Could you check a few things on this model? Use its own coordinates, in mm. A direction names the side the tool comes from. Round coordinates to 2 decimals unless told otherwise and drop trailing zeros. Loops run counter-clockwise (first coordinate to the right, second up) from the corner with the lowest first, then second, coordinate; pieces in that order, holes last. Notation, with made-up numbers: (68.25, -6) - (84.25, -6) arc R23 ccw to (84.25, 27) - close; hole circle Ø5 at (-36, -12.75). An arc over 180 degrees is marked (long way). Answer as CSV lines item,"result". Start each with the question number.
1) Suppose I cut it at D-D, the plane x = 17.05. Write out the boundary of the cut face in (y, z), then the cut area to 3 significant figures.
2) Please list where these lines run through material, in increasing order: line 1 along Y through (x, z) = (17.05, 9); line 2 along Y through (x, z) = (90.25, 10); line 3 along Y through (x, z) = (5, 11.5).
3) Which directions (+Z, -Z, +X, -X, +Y, -Y) give clear straight access to the entire face, cutting with the end or side of a thin tool? Please do faces 5 (the face through (48.31, 26.7, 7.28)), 6 (the face through (13, 13.25, 7)).
4) Suppose I cut it at A-A, the plane x = 90.25. Write out the boundary of the cut face in (y, z), then the cut area to 3 significant figures.
5) Suppose I cut it at C-C, the plane y = -27.5. Write out the boundary of the cut face in (x, z), then the cut area to 3 significant figures.
6) Suppose I cut it at B-B, the plane z = 9.5. Count the separate pieces of the cut face and the enclosed holes in it, then the cut area to 3 significant figures.
7) I'm going to push flat-ended pins straight in: pin 1 Ø1.5 at (x, z) = (23.5, 4.5) entering from +Y; pin 2 Ø2 at (x, z) = (27.5, 5.5) entering from +Y. Where does each tip first touch, or does it pass through?
8) We'd pull the mould along Y, two halves only. Please class faces 1 (the face through (13, -13.25, 7)), 2 (the face through (49.3, 37.215, 4.465)), 3 (the face through (0, 29, 7)), 4 (the face through (24, -12.2, 7.4)): pulls with the +Y half, pulls with the -Y half, needs draft (parallel to the pull), parting line crosses it, or undercut.
```python
from build123d import *

# Parameters (mm, degrees)
BOSS_EXTRUDE1_DEPTH         = 12.7
CHAMFER1_SIZE               = 5
FILLET1_R                   = 3.5
TAP_DRILL_FOR_M5X0_8_TAP1_D = 4.2
CUT_EXTRUDE1_DEPTH          = 2
CHAMFER3_SIZE               = 5
TAP_DRILL_FOR_M4X0_7_TAP1_D = 3.3
CUT_EXTRUDE2_DEPTH          = 2


with BuildPart() as part:
    # Sketch1 → Boss-Extrude1 (new body)
    with BuildSketch(Plane.XY):
        with BuildLine():
            Line((0, 38.75), (0, 13.25))
            Line((0, 13.25), (25, 13.25))
            Line((25, 13.25), (25, -13.25))
            Line((25, -13.25), (0, -13.25))
            Line((0, -13.25), (0, -38.75))
            ThreePointArc((0, -38.75), (0.292893219, -39.457106781), (1, -39.75))
            Line((1, -39.75), (99, -39.75))
            ThreePointArc((99, -39.75), (99.707106781, -39.457106781), (100, -38.75))
            Line((100, -38.75), (100, 38.75))
            ThreePointArc((100, 38.75), (99.707106781, 39.457106781), (99, 39.75))
            Line((99, 39.75), (1, 39.75))
            ThreePointArc((1, 39.75), (0.292893219, 39.457106781), (0, 38.75))
        make_face()
    extrude(amount=BOSS_EXTRUDE1_DEPTH)

    # Chamfer1
    chamfer1_edges = [part.edges().sort_by_distance(p)[0] for p in [
        (0, 13.25, 6.35),
        (0, -13.25, 6.35),
    ]]
    chamfer(chamfer1_edges, length=CHAMFER1_SIZE)

    # Fillet1
    fillet1_edges = [part.edges().sort_by_distance(p)[0] for p in [
        (25, -13.25, 6.35),
        (25, 13.25, 6.35),
    ]]
    fillet(fillet1_edges, radius=FILLET1_R)

    # Tap Drill for M5x0.8 Tap1 (through all)
    with Locations(Plane.XY.offset(12.7)):
        with Locations((10.25, 27.5), (50.25, 27.5), (90.25, 27.5), (90.25, -27.5), (50.25, -27.5), (10.25, -27.5)):
            Hole(TAP_DRILL_FOR_M5X0_8_TAP1_D / 2)

    # Sketch8 → Cut-Extrude1 (cut)
    with BuildSketch(Plane(origin=(0, 0, 0), x_dir=(-1, 0, 0), z_dir=(0, 0, -1))):
        with BuildLine():
            Line((-21.5, 13.25), (-5, 13.25))
            Line((-5, 13.25), (0, 18.25))
            Line((0, 18.25), (0, 38.75))
            ThreePointArc((0, 38.75), (-0.292893219, 39.457106781), (-1, 39.75))
            Line((-1, 39.75), (-99, 39.75))
            ThreePointArc((-99, 39.75), (-99.707106781, 39.457106781), (-100, 38.75))
            Line((-100, 38.75), (-100, -38.75))
            ThreePointArc((-100, -38.75), (-99.707106781, -39.457106781), (-99, -39.75))
            Line((-99, -39.75), (-1, -39.75))
            ThreePointArc((-1, -39.75), (-0.292893219, -39.457106781), (0, -38.75))
            Line((0, -38.75), (0, -18.25))
            Line((0, -18.25), (-5, -13.25))
            Line((-5, -13.25), (-21.5, -13.25))
            ThreePointArc((-21.5, -13.25), (-23.974873734, -12.224873734), (-25, -9.75))
            Line((-25, -9.75), (-25, 9.75))
            ThreePointArc((-25, 9.75), (-23.974873734, 12.224873734), (-21.5, 13.25))
        make_face()
        with BuildLine():
            Line((-84, -12.5), (-41, -12.5))
            ThreePointArc((-41, -12.5), (-38.525126266, -11.474873734), (-37.5, -9))
            Line((-37.5, -9), (-37.5, 9))
            ThreePointArc((-37.5, 9), (-38.525126266, 11.474873734), (-41, 12.5))
            Line((-41, 12.5), (-84, 12.5))
            ThreePointArc((-84, 12.5), (-86.474873734, 11.474873734), (-87.5, 9))
            Line((-87.5, 9), (-87.5, -9))
            ThreePointArc((-87.5, -9), (-86.474873734, -11.474873734), (-84, -12.5))
        make_face(mode=Mode.SUBTRACT)
    extrude(amount=-CUT_EXTRUDE1_DEPTH, mode=Mode.SUBTRACT)

    # Chamfer3
    # the kernel refuses this chamfer: 5 mm, written as the material it takes off along each edge
    with BuildSketch(Plane(origin=(111.85841494, -39.75, 2), x_dir=(0, 0.9996219169112968, -0.02749587661058636), z_dir=(-1, 0, 0)), Plane(origin=(-11.85841494, 39.75, 2), x_dir=(0, -0.9996219169112968, -0.02749587661058636), z_dir=(1, 0, 0))) as chamfer3_piece_1:
        Polygon((CHAMFER3_SIZE * 0.999621916911, -CHAMFER3_SIZE * 0.0274958766106), (-CHAMFER3_SIZE * 0.0274958766106, -CHAMFER3_SIZE * 0.999621916911), (0, 0), align=None)
    extrude(amount=123.71682988, mode=Mode.SUBTRACT)

    # Tap Drill for M4x0.7 Tap1 (through all)
    with Locations(Plane.XY.offset(12.7)):
        with Locations((17.05, 17.5), (17.05, -17.5), (49.05, -17.5), (49.05, 17.5)):
            Hole(TAP_DRILL_FOR_M4X0_7_TAP1_D / 2)

    # Sketch11 → Cut-Extrude2 (cut)
    with BuildSketch(Plane(origin=(0, 0, 0), x_dir=(-1, 0, 0), z_dir=(0, 0, -1))):
        with BuildLine():
            Line((-37.5, -9), (-37.5, 9))
            ThreePointArc((-37.5, 9), (-38.525126266, 11.474873734), (-41, 12.5))
            Line((-41, 12.5), (-84, 12.5))
            ThreePointArc((-84, 12.5), (-86.474873734, 11.474873734), (-87.5, 9))
            Line((-87.5, 9), (-87.5, -9))
            ThreePointArc((-87.5, -9), (-86.474873734, -11.474873734), (-84, -12.5))
            Line((-84, -12.5), (-41, -12.5))
            ThreePointArc((-41, -12.5), (-38.525126266, -11.474873734), (-37.5, -9))
        make_face()
    extrude(amount=-CUT_EXTRUDE2_DEPTH, mode=Mode.SUBTRACT)


solid = part.part
```
Filled sheet:
1,outline,"(-39.75, 7) - (-34.75, 2) - (-19.15, 2) - (-19.15, 12.7) - (-39.75, 12.7) - close; (-15.85, 2) - (-13.25, 2) - (-13.25, 12.7) - (-15.85, 12.7) - close; (13.25, 2) - (15.85, 2) - (15.85, 12.7) - (13.25, 12.7) - close; (19.15, 2) - (34.75, 2) - (39.75, 7) - (39.75, 12.7) - (19.15, 12.7) - close"
1,area,"471 mm²"
2,line 1,"-39.75 to -19.15, -15.85 to -13.25, 13.25 to 15.85, 19.15 to 39.75"
2,line 2,"-39.75 to -29.6, -25.4 to 25.4, 29.6 to 39.75"
2,line 3,"-39.75 to -13.25, 13.25 to 39.75"
3,face 5,"+Z, -Z"
3,face 6,"+Z, -Z, -X"
4,outline,"(-39.75, 7) - (-34.75, 2) - (-29.6, 2) - (-29.6, 12.7) - (-39.75, 12.7) - close; (-25.4, 2) - (25.4, 2) - (25.4, 12.7) - (-25.4, 12.7) - close; (29.6, 2) - (34.75, 2) - (39.75, 7) - (39.75, 12.7) - (29.6, 12.7) - close"
4,area,"736 mm²"
5,outline,"(0, 2) - (8.15, 2) - (8.15, 12.7) - (0, 12.7) - close; (12.35, 2) - (48.15, 2) - (48.15, 12.7) - (12.35, 12.7) - close; (52.35, 2) - (88.15, 2) - (88.15, 12.7) - (52.35, 12.7) - close; (92.35, 2) - (100, 2) - (100, 12.7) - (92.35, 12.7) - close"
5,area,"935 mm²"
6,separate pieces,"1"
6,enclosed holes,"10"
6,area,"7,150 mm²"
7,pin 1,"y = 38"
7,pin 2,"y = 39.25"
8,face 1,"undercut"
8,face 2,"pulls with the +Y half"
8,face 3,"needs draft"
8,face 4,"undercut"
